from build123d import *

# Parameters (mm, degrees)
F0_R     = 9.8806
F0_R_2   = 8.8265
F0_R_3   = 8.3566
F0_R_4   = 5.715
F0_R_5   = 7.8232
F0_R_6   = 6.8453
F0_R_7   = 6.4135
F0_R_8   = 5.8801
F0_R_9   = 6.3373
F1_DEPTH = 2.54
F2_DEPTH = 3.175
F3_DEPTH = 7.62
F4_DEPTH = 12.065
F5_DEPTH = 12.7
F6_R     = 3.937
F6_R_2   = 2.7305
F6_R_3   = 2.286
F6_R_4   = 1.8415
F6_R_5   = 1.3335
F6_R_6   = 2.032
F7_DEPTH = 25.4
F9_DEPTH = 25.4


with BuildPart() as f1:
    # F0 (on Top) → F1 (new body)
    with BuildSketch(Plane.XY):
        Polygon((-61.88075, 12.7), (-71.05015, 12.7), (-71.05015, -12.7), (-61.88075, -12.7), (-61.88075, -41.906793621), (71.05015, -32.2915386482), (71.05015, 32.2915386482), (-61.88075, 41.906793621), align=None)
        with Locations((-45.65015, -24.4856)):
            Circle(F0_R, mode=Mode.SUBTRACT)
        with Locations((-23.76805, -23.9338478505)):
            Circle(F0_R_2, mode=Mode.SUBTRACT)
        with Locations((-3.94335, -22.9710008273)):
            Circle(F0_R_3, mode=Mode.SUBTRACT)
        with Locations((-34.18205, -8.89)):
            Circle(F0_R_4, mode=Mode.SUBTRACT)
        with Locations((-13.84935, -8.89)):
            Circle(F0_R_4, mode=Mode.SUBTRACT)
        with Locations((13.90015, -22.2151253099)):
            Circle(F0_R_5, mode=Mode.SUBTRACT)
        with Locations((30.25775, -22.0123902971)):
            Circle(F0_R_6, mode=Mode.SUBTRACT)
        with Locations((45.65015, -21.3487)):
            Circle(F0_R_7, mode=Mode.SUBTRACT)
        with Locations((4.98475, -9.0551)):
            Circle(F0_R_8, mode=Mode.SUBTRACT)
        with Locations((22.07895, -9.0551)):
            Circle(F0_R_8, mode=Mode.SUBTRACT)
        with Locations((37.95395, -9.0551)):
            Circle(F0_R_8, mode=Mode.SUBTRACT)
        with Locations((-46.88205, 0)):
            Circle(F0_R_8, mode=Mode.SUBTRACT)
        with Locations((-34.18205, 8.89)):
            Circle(F0_R_4, mode=Mode.SUBTRACT)
        with Locations((-13.84935, 8.89)):
            Circle(F0_R_4, mode=Mode.SUBTRACT)
        with Locations((-45.65015, 24.4856)):
            Circle(F0_R, mode=Mode.SUBTRACT)
        with Locations((-23.76805, 23.9338478505)):
            Circle(F0_R_2, mode=Mode.SUBTRACT)
        with Locations((-3.94335, 23.5057943876)):
            Circle(F0_R_5, mode=Mode.SUBTRACT)
        with Locations((4.98475, 8.89)):
            Circle(F0_R_4, mode=Mode.SUBTRACT)
        with Locations((22.07895, 8.89)):
            Circle(F0_R_4, mode=Mode.SUBTRACT)
        with Locations((37.95395, 9.0551)):
            Circle(F0_R_8, mode=Mode.SUBTRACT)
        with Locations((13.90015, 23.1955801706)):
            Circle(F0_R_6, mode=Mode.SUBTRACT)
        with Locations((30.25775, 22.5217174975)):
            Circle(F0_R_9, mode=Mode.SUBTRACT)
        with Locations((45.65015, 21.8821)):
            Circle(F0_R_8, mode=Mode.SUBTRACT)
        with Locations((-45.65015, 24.4856)):
            Circle(F0_R)
        with Locations((-45.65015, -24.4856)):
            Circle(F0_R)
        with Locations((-23.76805, 23.9338478505)):
            Circle(F0_R_2)
        with Locations((-23.76805, -23.9338478505)):
            Circle(F0_R_2)
        with Locations((-3.94335, -22.9710008273)):
            Circle(F0_R_3)
        with Locations((-3.94335, 23.5057943876)):
            Circle(F0_R_5)
        with Locations((13.90015, -22.2151253099)):
            Circle(F0_R_5)
        with Locations((13.90015, 23.1955801706)):
            Circle(F0_R_6)
        with Locations((30.25775, -22.0123902971)):
            Circle(F0_R_6)
        with Locations((45.65015, -21.3487)):
            Circle(F0_R_7)
        with Locations((30.25775, 22.5217174975)):
            Circle(F0_R_9)
        with Locations((45.65015, 21.8821)):
            Circle(F0_R_8)
        with Locations((37.95395, 9.0551)):
            Circle(F0_R_8)
        with Locations((-46.88205, 0)):
            Circle(F0_R_8)
        with Locations((4.98475, -9.0551)):
            Circle(F0_R_8)
        with Locations((22.07895, -9.0551)):
            Circle(F0_R_8)
        with Locations((37.95395, -9.0551)):
            Circle(F0_R_8)
        with Locations((22.07895, 8.89)):
            Circle(F0_R_4)
        with Locations((4.98475, 8.89)):
            Circle(F0_R_4)
        with Locations((-13.84935, 8.89)):
            Circle(F0_R_4)
        with Locations((-34.18205, 8.89)):
            Circle(F0_R_4)
        with Locations((-34.18205, -8.89)):
            Circle(F0_R_4)
        with Locations((-13.84935, -8.89)):
            Circle(F0_R_4)
    extrude(amount=F1_DEPTH)

    # F0 (on Top) → F2 (join)
    with BuildSketch(Plane.XY):
        with Locations((-23.76805, 23.9338478505)):
            Circle(F0_R_2)
        with Locations((-23.76805, -23.9338478505)):
            Circle(F0_R_2)
    extrude(amount=F2_DEPTH)

    # F0 (on Top) → F3 (join)
    with BuildSketch(Plane.XY):
        with Locations((-3.94335, 23.5057943876)):
            Circle(F0_R_5)
        with Locations((-3.94335, -22.9710008273)):
            Circle(F0_R_3)
        with Locations((13.90015, -22.2151253099)):
            Circle(F0_R_5)
    extrude(amount=F3_DEPTH)

    # F0 (on Top) → F4 (join)
    with BuildSketch(Plane.XY):
        with Locations((13.90015, 23.1955801706)):
            Circle(F0_R_6)
        with Locations((30.25775, 22.5217174975)):
            Circle(F0_R_9)
        with Locations((45.65015, 21.8821)):
            Circle(F0_R_8)
        with Locations((30.25775, -22.0123902971)):
            Circle(F0_R_6)
        with Locations((45.65015, -21.3487)):
            Circle(F0_R_7)
        with Locations((37.95395, -9.0551)):
            Circle(F0_R_8)
        with Locations((22.07895, -9.0551)):
            Circle(F0_R_8)
        with Locations((37.95395, 9.0551)):
            Circle(F0_R_8)
        with Locations((-46.88205, 0)):
            Circle(F0_R_8)
    extrude(amount=F4_DEPTH)

    # F0 (on Top) → F5 (join)
    with BuildSketch(Plane.XY):
        with Locations((-13.84935, 8.89)):
            Circle(F0_R_4)
        with Locations((4.98475, 8.89)):
            Circle(F0_R_4)
        with Locations((22.07895, 8.89)):
            Circle(F0_R_4)
        with Locations((4.98475, -9.0551)):
            Circle(F0_R_8)
        with Locations((-13.84935, -8.89)):
            Circle(F0_R_4)
        with Locations((-34.18205, -8.89)):
            Circle(F0_R_4)
        with Locations((-34.18205, 8.89)):
            Circle(F0_R_4)
    extrude(amount=F5_DEPTH)

    # F6 (on face) → F7 (join)
    with BuildSketch(Plane.XY.offset(2.54)):
        with Locations((-45.65015, 24.4856)):
            Circle(F6_R)
        with Locations((-23.76805, 23.9338478505)):
            Circle(F6_R)
        with Locations((-3.94335, 23.5057943876)):
            Circle(F6_R_2)
        with Locations((13.90015, 23.1955801706)):
            Circle(F6_R_2)
        with Locations((30.25775, 22.5217174975)):
            Circle(F6_R_3)
        with Locations((45.65015, 21.8821)):
            Circle(F6_R_3)
        with Locations((37.95395, 9.0551)):
            Circle(F6_R_3)
        with Locations((22.07895, 8.89)):
            Circle(F6_R_4)
        with Locations((4.98475, 8.89)):
            Circle(F6_R_4)
        with Locations((-13.84935, 8.89)):
            Circle(F6_R_5)
        with Locations((-34.18205, 8.89)):
            Circle(F6_R_5)
        with Locations((-45.65015, -24.4856)):
            Circle(F6_R)
        with Locations((-23.76805, -23.9338478505)):
            Circle(F6_R)
        with Locations((-3.94335, -22.9710008273)):
            Circle(F6_R_2)
        with Locations((13.90015, -22.2151253099)):
            Circle(F6_R_2)
        with Locations((30.25775, -22.0123902971)):
            Circle(F6_R_2)
        with Locations((45.65015, -21.3487)):
            Circle(F6_R_3)
        with Locations((37.95395, -9.0551)):
            Circle(F6_R_3)
        with Locations((22.07895, -9.0551)):
            Circle(F6_R_3)
        with Locations((4.98475, -9.0551)):
            Circle(F6_R_6)
        with Locations((-13.84935, -8.89)):
            Circle(F6_R_6)
        with Locations((-34.18205, -8.89)):
            Circle(F6_R_5)
        with Locations((-46.88205, 0)):
            Circle(F6_R_3)
    extrude(amount=F7_DEPTH)

    # F8 (on face) → F9 (join, through all)
    with BuildSketch(Plane.XZ.offset(12.7)):
        with BuildLine():
            Line((-71.05015, 6.35), (-71.05015, 2.54))
            Line((-71.05015, 2.54), (-69.76745, 2.54))
            Line((-69.76745, 2.54), (-69.76745, 6.35))
            ThreePointArc((-69.76745, 6.35), (-66.46545, 9.652), (-63.16345, 6.35))
            Line((-63.16345, 6.35), (-63.16345, 2.54))
            Line((-63.16345, 2.54), (-61.88075, 2.54))
            Line((-61.88075, 2.54), (-61.88075, 6.35))
            ThreePointArc((-61.88075, 6.35), (-66.46545, 10.9347), (-71.05015, 6.35))
        make_face()
    extrude(amount=-F9_DEPTH)


solid = f1.part
CAD build for the part. Positions are in the model's coordinates, mm. A direction names the side the tool comes from. Give positions to 0.01 mm unless a question says otherwise; leave off trailing zeros. Loops run counter-clockwise (first coordinate to the right, second up) from the corner with the lowest first, then second, coordinate; pieces in that order, holes last. Notation, with made-up numbers: M 45,-9.75 L 66,-9.75 A17 ccw 66,4.25 Z; hole C -20,53.5 d11. An arc over 180 degrees is marked long. One line per question, with ' | ' between items. Start each with the question number.
1. Saw through at D-D on x = -18. Give the cut face in (y, z) (3 decimals), plus the area to 3 significant figures.
2. Two-plate mould, pull along X, no slides. Class faces 4 (the face through (-14, -9, 27.94)), 5 (the face through (4.219, -3.225, 7.549)), 6 (the face through (71.05, 0, 1)): pulls with the +X half, pulls with the -X half, needs draft (parallel to the pull), parting line crosses it, or undercut.
3. Saw through at B-B on z = 18.5. State how many separate pieces and enclosed holes the cut face has, plus the area to 3 significant figures.
4. Probe L1, parallel to X at y = -23, z = 16.5; L2, parallel to X at y = -12, z = 10; L3, parallel to X at y = 9.5, z = 20.75. List the from-to ranges inside material, lowest first. Write a range as from..to.
5. 3-axis set-ups, long thin cutter, end or side, ignore diameter. For faces 1 (the face through (21.362, -19.865, 5.044)), 2 (the face through (3.654, -37.166, 1.252)), 3 (the face through (-66.54, -0.18, 9.65)): which of +Z, -Z, +X, -X, +Y, -Y reach the whole face in a straight line?
6. Saw through at A-A on y = 0. Give the cut face in (x, z) (3 decimals), plus the area to 3 significant figures.
7. Saw through at C-C on x = 50. Give the cut face in (y, z) (3 decimals).
8. Flat gauge pins, fed straight in: pin 1 (10 mm diameter, centred on y = 10, z = 20, fed in from -X); pin 2 (6 mm diameter, centred on y = 1.5, z = 18.5, fed in from +X); pin 3 (5.5 mm diameter, centred on x = -11.5, y = -10.5, fed in from +Z); pin 4 (4 mm diameter, centred on x = 7.5, z = 20.5, fed in from +Y). Where does each tip first touch, or does it go through?
Result sheet:
1) outline: M -38.733,0 L 38.733,0 L 38.733,2.54 L 30.615,2.54 L 30.615,3.175 L 17.253,3.175 L 17.253,2.54 L 12.819,2.54 L 12.819,12.7 L 4.961,12.7 L 4.961,2.54 L -4.961,2.54 L -4.961,12.7 L -12.819,12.7 L -12.819,2.54 L -17.253,2.54 L -17.253,3.175 L -30.615,3.175 L -30.615,2.54 L -38.733,2.54 Z | area: 373 mm^2
2) face 4: needs draft | face 5: undercut | face 6: pulls with the +X half
3) separate pieces: 23 | enclosed holes: 0 | area: 491 mm^2
4) L1: x = -49.3..-42, -27.59..-19.94, -6.67..-1.21, 11.28..16.52, 27.71..32.8, 44.07..47.23 | L2: x = -69.24..-63.69, -38.98..-29.39, -18.64..-9.05, -0.1..10.07, 16.99..27.17, 32.86..43.04 | L3: x = -35.37..-33, -15.04..-12.66, 3.25..6.72, 20.34..23.82, 35.71..40.2
5) face 1: +Z | face 2: +Z, -Z, +X, -Y | face 3: +Y, -Y
6) outline: M -71.05,0 L 71.05,0 L 71.05,2.54 L -41.002,2.54 L -41.002,12.065 L -44.596,12.065 L -44.596,27.94 L -49.168,27.94 L -49.168,12.065 L -52.762,12.065 L -52.762,2.54 L -61.881,2.54 L -61.881,6.35 A4.585 ccw -71.05,6.35 Z; hole M -69.767,2.54 L -63.163,2.54 L -63.163,6.35 A3.302 ccw -69.767,6.35 Z | area: 571 mm^2
7) outline: M -33.814,0 L 33.814,0 L 33.814,2.54 L 25.839,2.54 L 25.839,12.065 L 17.926,12.065 L 17.926,2.54 L -16.636,2.54 L -16.636,12.065 L -26.062,12.065 L -26.062,2.54 L -33.814,2.54 Z
8) pin 1: stops at x = -35.52 | pin 2: stops at x = -44.6 | pin 3: stops at z = 27.94 | pin 4: stops at y = 10.66
